For this review, take the finished solid that the model builds, in its own axes (mm). Face numbers are marked on the shaded views. A direction names the side the tool comes from. Round coordinates to 2 decimals unless told otherwise and drop trailing zeros. Order: outer loops, then holes, each group sorted by start corner. A loop starts at its lowest first (then second) coordinate and runs counter-clockwise, first axis right, second up. Notation, with made-up numbers: (76, 56) -> (126, 56) arc R15 cw to (126, 69) -> close; hole circle Ø2 at (23.5, 41.5). An arc over 180 degrees is marked (long way). Use a Markdown table: item, result. Add a question column.
1) Wall thickness on line 1 along Z through (x, y) = (-11.75, 0); line 2 along X through (y, z) = (3.25, -0.75); line 3 along X through (y, z) = (-0.5, -3.25): over which ranges is each line inside the solid? List them lowest first. Write a range as [from, to].
2) Clearance check with flat-ended pins moving along their axes: P1, Ø3, axis at y = 0, z = 0, coming from the -X side; P2, Ø2, axis at y = -1.5, z = 1, coming from the -X side; P3, Ø2, axis at x = -10.5, y = -1.5, coming from the +Z side; P4, Ø4, axis at x = -12, z = -3, coming from the -Y side. State where each tip first meets the part, or that it passes through.
3) Draft analysis for pull direction X (two halves, no side actions). For the marked faces 4, 5 and 6, state which applies: pulls with the +X half, pulls with the -X half, needs draft (parallel to the pull), parting line crosses it, or undercut.
4) Consider section B-B (x = 4.5). State the section outline as (y, z) points, plus the area to 3 significant figures.
5) Consider section A-A (x = -3.75). State the section outline as (y, z) points, plus the area to 3 significant figures.
6) Machinability: for the marked faces 1, 2 and 3, which of the approach directions +Z, -Z, +X, -X, +Y, -Y give a long, thin tool a straight path to every point of the face, cutting with its end or side? Answer none if there is none.
```python
from build123d import *

# Parameters (mm, degrees)
CORTE_EXTRUS_O1_REACH = 20
FILETE1_R             = 0.25
FILETE2_R             = 0.25
CHANFRO1_SIZE         = 0.3


with BuildPart() as part:
    # Esboço1 → Revolução1 (revolve)
    with BuildSketch(Plane.XY):
        Polygon((-13.322649731, 3), (-13.122649731, 3), (-12.833974596, 3.5), (-12.433974596, 3.5), (-12.145299462, 3), (-2.5, 3), (-2.5, 4), (3.5, 4), (3.5, 2.25), (7.5, 2.25), (7.5, 1.75), (-9.200961894, 1.75), (-10.5, 2.5), (-14.5, 2.5), (-14.5, 3), (-14.3, 3), (-14.011324865, 3.5), (-13.611324865, 3.5), align=None)
    revolve(axis=Axis((-29.721905334, 0, 0), (1, 0, 0)))

    # Esboço2 → Corte-extrusão1 (cut, up to next)
    with BuildSketch(Plane(origin=(3.5, 0, 0), x_dir=(0, 0, -1), z_dir=(1, 0, 0)), mode=Mode.PRIVATE) as corte_extrus_o1_sk1:
        with BuildLine():
            Line((-2, 3.464101615), (2, 3.464101615))
            ThreePointArc((2, 3.464101615), (0, 4), (-2, 3.464101615))
        make_face()
    corte_extrus_o1_tool1 = extrude(corte_extrus_o1_sk1.sketch, amount=-CORTE_EXTRUS_O1_REACH, mode=Mode.PRIVATE) & part.part
    add(corte_extrus_o1_tool1.solids().sort_by_distance((3.5, 3.679741, 0))[0], mode=Mode.SUBTRACT)
    # Esboço2 → Corte-extrusão1 (cut, up to next)
    with BuildSketch(Plane(origin=(3.5, 0, 0), x_dir=(0, 0, -1), z_dir=(1, 0, 0)), mode=Mode.PRIVATE) as corte_extrus_o1_sk2:
        with BuildLine():
            Line((-4, 0), (-2, 3.464101615))
            ThreePointArc((-2, 3.464101615), (-3.464101615, 2), (-4, 0))
        make_face()
    corte_extrus_o1_tool2 = extrude(corte_extrus_o1_sk2.sketch, amount=-CORTE_EXTRUS_O1_REACH, mode=Mode.PRIVATE) & part.part
    add(corte_extrus_o1_tool2.solids().sort_by_distance((3.5, 1.839871, 3.18675))[0], mode=Mode.SUBTRACT)
    # Esboço2 → Corte-extrusão1 (cut, up to next)
    with BuildSketch(Plane(origin=(3.5, 0, 0), x_dir=(0, 0, -1), z_dir=(1, 0, 0)), mode=Mode.PRIVATE) as corte_extrus_o1_sk3:
        with BuildLine():
            ThreePointArc((-4, 0), (-3.464101615, -2), (-2, -3.464101615))
            Line((-2, -3.464101615), (-4, 0))
        make_face()
    corte_extrus_o1_tool3 = extrude(corte_extrus_o1_sk3.sketch, amount=-CORTE_EXTRUS_O1_REACH, mode=Mode.PRIVATE) & part.part
    add(corte_extrus_o1_tool3.solids().sort_by_distance((3.5, -1.839871, 3.18675))[0], mode=Mode.SUBTRACT)
    # Esboço2 → Corte-extrusão1 (cut, up to next)
    with BuildSketch(Plane(origin=(3.5, 0, 0), x_dir=(0, 0, -1), z_dir=(1, 0, 0)), mode=Mode.PRIVATE) as corte_extrus_o1_sk4:
        with BuildLine():
            ThreePointArc((-2, -3.464101615), (0, -4), (2, -3.464101615))
            Line((2, -3.464101615), (-2, -3.464101615))
        make_face()
    corte_extrus_o1_tool4 = extrude(corte_extrus_o1_sk4.sketch, amount=-CORTE_EXTRUS_O1_REACH, mode=Mode.PRIVATE) & part.part
    add(corte_extrus_o1_tool4.solids().sort_by_distance((3.5, -3.679741, 0))[0], mode=Mode.SUBTRACT)
    # Esboço2 → Corte-extrusão1 (cut, up to next)
    with BuildSketch(Plane(origin=(3.5, 0, 0), x_dir=(0, 0, -1), z_dir=(1, 0, 0)), mode=Mode.PRIVATE) as corte_extrus_o1_sk5:
        with BuildLine():
            ThreePointArc((2, -3.464101615), (3.464101615, -2), (4, 0))
            Line((4, 0), (2, -3.464101615))
        make_face()
    corte_extrus_o1_tool5 = extrude(corte_extrus_o1_sk5.sketch, amount=-CORTE_EXTRUS_O1_REACH, mode=Mode.PRIVATE) & part.part
    add(corte_extrus_o1_tool5.solids().sort_by_distance((3.5, -1.839871, -3.18675))[0], mode=Mode.SUBTRACT)
    # Esboço2 → Corte-extrusão1 (cut, up to next)
    with BuildSketch(Plane(origin=(3.5, 0, 0), x_dir=(0, 0, -1), z_dir=(1, 0, 0)), mode=Mode.PRIVATE) as corte_extrus_o1_sk6:
        with BuildLine():
            Line((2, 3.464101615), (4, 0))
            ThreePointArc((4, 0), (3.464101615, 2), (2, 3.464101615))
        make_face()
    corte_extrus_o1_tool6 = extrude(corte_extrus_o1_sk6.sketch, amount=-CORTE_EXTRUS_O1_REACH, mode=Mode.PRIVATE) & part.part
    add(corte_extrus_o1_tool6.solids().sort_by_distance((3.5, 1.839871, -3.18675))[0], mode=Mode.SUBTRACT)

    # Filete1
    filete1_edges = [part.edges().sort_by_distance(p)[0] for p in [
        (-14.011324865, -3.5, 0),
        (-13.611324865, -3.5, 0),
    ]]
    fillet(filete1_edges, radius=FILETE1_R)

    # Filete2
    filete2_edges = [part.edges().sort_by_distance(p)[0] for p in [
        (-12.833974596, -3.5, 0),
        (-12.433974596, -3.5, 0),
    ]]
    fillet(filete2_edges, radius=FILETE2_R)

    # Chanfro1
    chanfro1_edges = [part.edges().sort_by_distance(p)[0] for p in [
        (7.5, -1.75, 0),
    ]]
    chamfer(chanfro1_edges, length=CHANFRO1_SIZE)


solid = part.part
```
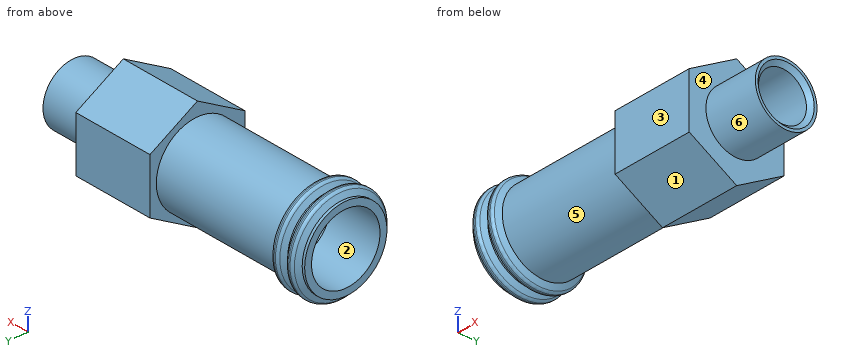
Results list:
| question | item | result |
|---|---|---|
| 1 | line 1 | [-3, -2.5], [2.5, 3] |
| 1 | line 2 | [-14.11, -13.52], [-12.93, -12.34], [-2.5, 3.5] |
| 1 | line 3 | [-14.13, -13.49], [-12.96, -12.31], [-2.5, 3.5] |
| 2 | P1 | through |
| 2 | P2 | x = -14.5 |
| 2 | P3 | z = 2.96 |
| 2 | P4 | y = -3.33 |
| 3 | face 4 | pulls with the +X half |
| 3 | face 5 | undercut |
| 3 | face 6 | needs draft |
| 4 | outline | circle Ø4.5 at (0, 0); hole circle Ø3.5 at (0, 0) |
| 4 | area | 6.28 mm2 |
| 5 | outline | circle Ø6 at (0, 0); hole circle Ø3.5 at (0, 0) |
| 5 | area | 18.7 mm2 |
| 6 | face 1 | -Z, +X, -Y |
| 6 | face 2 | -X |
| 6 | face 3 | +Z, -Z, +X, -Y |
